Check sheet for the drawn part. Datum: minimum x, y, z corner. Units: mm. Round coordinates to 2 decimals unless told otherwise and drop trailing zeros. Write each loop counter-clockwise with the first axis right and the second up, starting at its lowest first coordinate (ties: lowest second). Pieces come first, ordered by that corner, then holes. Notation, with made-up numbers: (56, 57.25) - (99, 57.25) arc R18 cw to (99, 64.25) - close; hole circle Ø5 at (-37, 24). An arc over 180 degrees is marked (long way). Answer as a JSON object with one key per item and string values.
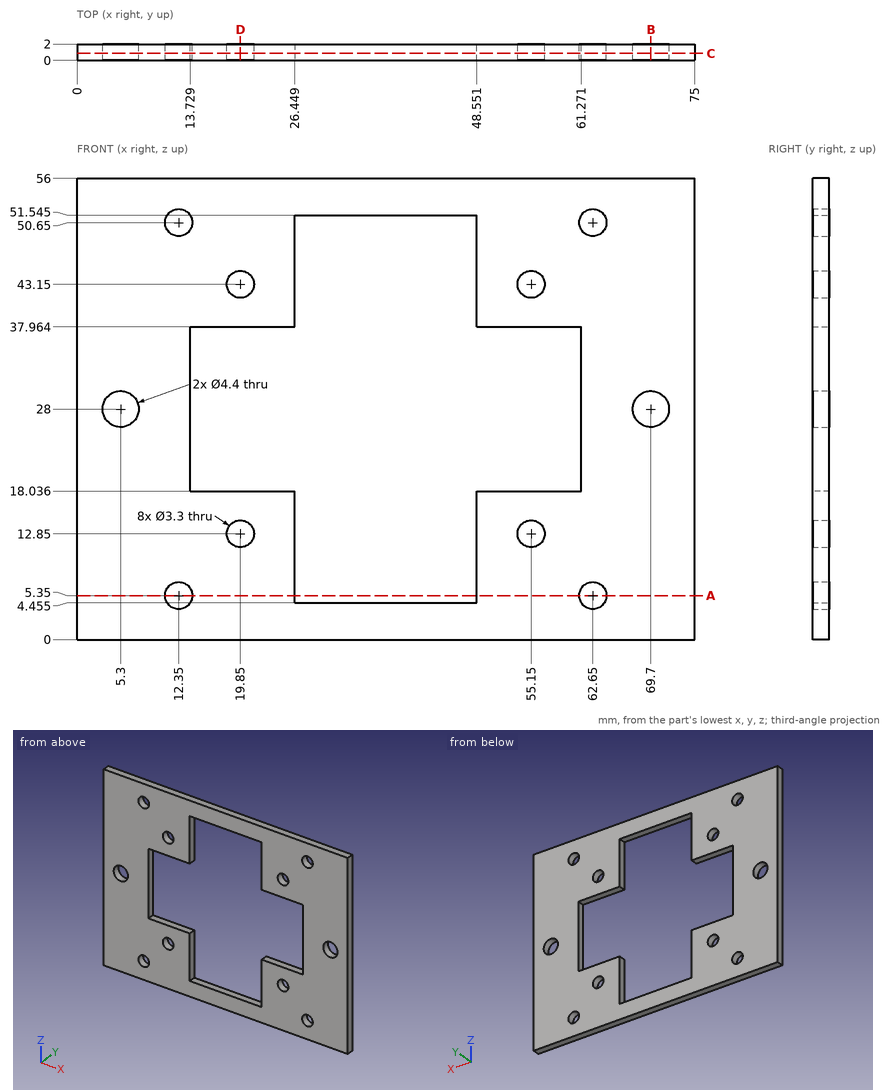
Q1. Section check C-C, the plane y = 0.85. State how many separate pieces and enclosed holes the cut face has, then the cut area to 3 significant figures.
Geometry check:
{"separate pieces": "1", "enclosed holes": "11", "area": "2,550 mm2"}
Q2. Section check B-B, the plane x = 69.7. Record the cut outline in (y, z).
Geometry check:
{"outline": "(0, 0) - (2, 0) - (2, 25.8) - (0, 25.8) - close; (0, 30.2) - (2, 30.2) - (2, 56) - (0, 56) - close"}
Q3. Gauge pin test, flat end, axial feed: P1, Ø2.5, axis at x = 55.15, z = 43.15, coming from the -Y side. Record the tip position at first contact, or that the pin passes through.
Geometry check:
{"P1": "passes through"}
Q4. Section check A-A, the plane z = 5.35. Record the cut outline in (x, y).
Geometry check:
{"outline": "(0, 0) - (10.7, 0) - (10.7, 2) - (0, 2) - close; (14, 0) - (26.45, 0) - (26.45, 2) - (14, 2) - close; (48.55, 0) - (61, 0) - (61, 2) - (48.55, 2) - close; (64.3, 0) - (75, 0) - (75, 2) - (64.3, 2) - close"}
Q5. Material ranges on line 1 along Z through (x, y) = (12.35, 0.5); line 2 along Z through (x, y) = (19.85, 0.4); line 3 along Z through (x, y) = (69.7, 0.75), recorded low to high. Write a range as [from, to].
Geometry check:
{"line 1": "z = [0, 3.7], [7, 49], [52.3, 56]", "line 2": "z = [0, 11.2], [14.5, 18.04], [37.96, 41.5], [44.8, 56]", "line 3": "z = [0, 25.8], [30.2, 56]"}
Q6. Section check D-D, the plane x = 19.85. Record the cut outline in (y, z).
Geometry check:
{"outline": "(0, 0) - (2, 0) - (2, 11.2) - (0, 11.2) - close; (0, 14.5) - (2, 14.5) - (2, 18.04) - (0, 18.04) - close; (0, 37.96) - (2, 37.96) - (2, 41.5) - (0, 41.5) - close; (0, 44.8) - (2, 44.8) - (2, 56) - (0, 56) - close"}
